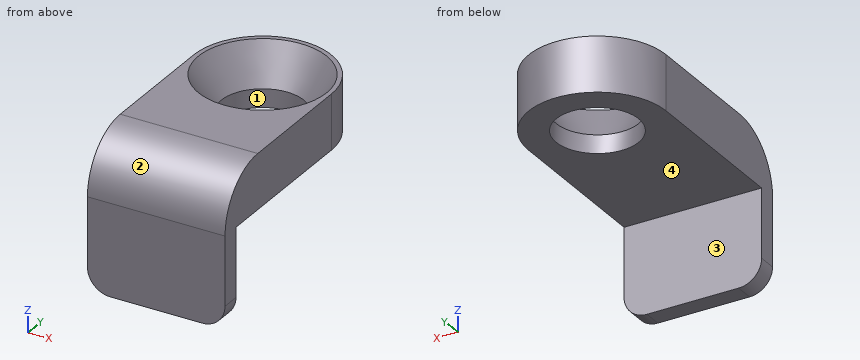
```python
from build123d import *

# Parameters (mm, degrees)
F0_R     = 12
F0_W     = 30
F0_H     = 4
F0_R_2   = 9
F1_DEPTH = 3
F2_DEPTH = 20
F3_DEPTH = 6
F4_SIZE  = 2.99999
F6_DEPTH = 12
F7_SIZE2 = 5
F7_SIZE  = 8
F8_DEPTH = 4
F9_R     = 12
F10_R    = 5


# Not quite as in the source:
# - a fillet or chamfer is up to 0.001 mm smaller than in the source, because OpenCascade refuses the exact size


with BuildPart() as f1:
    # F0 (on Top) → F1 (new body)
    with BuildSketch(Plane.XY):
        with BuildLine():
            Line((15, -35), (15, 0))
            ThreePointArc((15, 0), (0, 15), (-15, 0))
            Line((-15, 0), (-15, -35))
            Line((-15, -35), (15, -35))
        make_face()
        Circle(F0_R, mode=Mode.SUBTRACT)
        with Locations((0, -37)):
            Rectangle(F0_W, F0_H)
        Circle(F0_R)
        Circle(F0_R_2, mode=Mode.SUBTRACT)
    extrude(amount=F1_DEPTH)

    # F0 (on Top) → F2 (join)
    with BuildSketch(Plane.XY):
        with Locations((0, -37)):
            Rectangle(F0_W, F0_H)
    extrude(amount=-F2_DEPTH)

    # F0 (on Top) → F3 (join)
    with BuildSketch(Plane.XY):
        Circle(F0_R)
        Circle(F0_R_2, mode=Mode.SUBTRACT)
    extrude(amount=F3_DEPTH)

    # F4 (size 3 in the source; OpenCascade refuses exactly that, so slightly less here)
    f4_edges = [f1.edges().sort_by_distance(p)[0] for p in [
        (-12, 0, 3),
    ]]
    chamfer(f4_edges, length=F4_SIZE)

    # F0 (on Top) → F6 (join)
    with BuildSketch(Plane.XY):
        with BuildLine():
            Line((15, -35), (15, 0))
            ThreePointArc((15, 0), (0, 15), (-15, 0))
            Line((-15, 0), (-15, -35))
            Line((-15, -35), (15, -35))
        make_face()
        Circle(F0_R, mode=Mode.SUBTRACT)
        Circle(F0_R)
        Circle(F0_R_2, mode=Mode.SUBTRACT)
    extrude(amount=F6_DEPTH)

    # F7
    f7_edges = [f1.edges().sort_by_distance(p)[0] for p in [
        (-9, 0, 12),
    ]]
    f7_side = f1.faces().sort_by_distance((-9, 0, 6))[0]
    chamfer(f7_edges, length=F7_SIZE, length2=F7_SIZE2, reference=f7_side)

    # F8 (add, through all): a face of the model
    f8_faces = [f1.faces().sort_by_distance(p)[0] for p in [
        (0, -35, 7.5),
    ]]
    extrude(f8_faces, amount=F8_DEPTH)

    # F9
    f9_edges = [f1.edges().sort_by_distance(p)[0] for p in [
        (0, -39, 12),
    ]]
    fillet(f9_edges, radius=F9_R)

    # F10
    f10_edges = [f1.edges().sort_by_distance(p)[0] for p in [
        (-15, -37, -20),
        (15, -37, -20),
    ]]
    fillet(f10_edges, radius=F10_R)


solid = f1.part
```
Source: CAD feature listing. Evaluate the final solid. Frame: model axes, mm. Face numbers are marked on the shaded views. Give positions to 0.01 mm unless a question says otherwise; leave off trailing zeros. Loops run counter-clockwise (first coordinate to the right, second up) from the corner with the lowest first, then second, coordinate; pieces in that order, holes last. Notation, with made-up numbers: (80, 48) -> (118, 48) arc R18 ccw to (118, 60) -> close; hole circle Ø6 at (67.25, 7.25). An arc over 180 degrees is marked (long way). Put each result on its own line as item: value. Start each with the question number.
1) Cut plane B-B (z = -3). Return loops of the section in (x, y), then the cut area to 3 significant figures.
2) Cut plane A-A (x = 0). Return loops of the section in (y, z).
3) Cut plane D-D (y = -32.5). Return loops of the section in (x, z).
4) Cut plane C-C (z = 9). Return loops of the section in (x, y) (3 decimals), then the cut area to 3 significant figures.
5) Draft query along Y for the marked faces 1, 2, 3 and 4. Return one class per face: released by +Y, released by -Y, zero draft, split by the parting line, or undercut.
6) Material intervals for probe 1 along Z at (x, y) = (7.25, -16.5); probe 2 along Y at (x, z) = (9.25, -14); probe 3 along Y at (x, z) = (0, 2.55), sorted ascending.
7) Contact query for flat-ended pins moving along their axis: P1, Ø14.5, axis at x = 0, y = 0, coming from the -Z side; P2, Ø2, axis at x = -11.5, z = 4.5, coming from the +Y side; P3, Ø6, axis at x = -7.5, y = 7, coming from the +Z side; P4, Ø1, axis at x = 1, y = -16.5, coming from the -Z side. Output: stop coordinate, or through.
Results are:
1. outline: (-15, -39) -> (15, -39) -> (15, -35) -> (-15, -35) -> close
1. area: 120 mm2
2. outline: (-39, -20) -> (-35, -20) -> (-35, 0) -> (-9, 0) -> (-9, 4) -> (-14, 12) -> (-27, 12) arc R12 ccw to (-39, 0) -> close; (9, 0) -> (15, 0) -> (15, 12) -> (14, 12) -> (9, 4) -> close
3. outline: (-15, 0) -> (15, 0) -> (15, 10.67) -> (-15, 10.67) -> close
4. outline: (-15, -34.937) -> (15, -34.937) -> (15, 0) arc R15 ccw to (-15, 0) -> close; hole circle Ø24.25 at (0, 0)
4. area: 940 mm2
5. face 1: undercut
5. face 2: released by -Y
5. face 3: released by +Y
5. face 4: zero draft
6. probe 1: z = 0 to 12
6. probe 2: y = -39 to -35
6. probe 3: y = -38.73 to -9, 9 to 15
7. P1: passes through
7. P2: stops at y = 10.71
7. P3: stops at z = 10.81
7. P4: stops at z = 0
